Verification items for the finished model (mm, model axes). A direction names the side the tool comes from. Give positions to 0.01 mm unless a question says otherwise; leave off trailing zeros. Write each loop counter-clockwise with the first axis right and the second up, starting at its lowest first coordinate (ties: lowest second). Pieces come first, ordered by that corner, then holes.
from build123d import *

# Parameters (mm, degrees)
SKETCH1_W                       = 8
SKETCH1_H                       = 15
FIRST_CHAMBER_BLOCK_DEPTH       = 15
SKETCH2_W                       = 6
SKETCH2_H                       = 11
FIRST_CHAMBER_CAVITY_DEPTH      = 13
SKETCH3_W                       = 15
SKETCH3_H                       = 3
CHAMBER_SPACER_DEPTH            = 2
PATTERN_CHAMBERS_COUNT          = 11
PATTERN_CHAMBERS_PITCH          = 10
SKETCH4_W                       = 15
SKETCH4_H                       = 12
THICKEN_END_1_DEPTH             = 2
SKETCH5_W                       = 15
SKETCH5_H                       = 15
THICKEN_END_2_DEPTH             = 2
SKETCH6_W                       = 94
SKETCH6_H                       = 2
CENTRAL_AIR_CHANNEL_DEPTH       = 2
SKETCH7_W                       = 108
SKETCH7_H                       = 13
SKETCH7_W_2                     = 106
SKETCH7_H_2                     = 11
BONDING_RIDGE_DEPTH             = 2
SKETCH9_W                       = 2
SKETCH9_H                       = 2.5
BONDING_BUMPS_DEPTH             = 2
PATTERN_BONDING_BUMPS_COUNT     = 10
PATTERN_BONDING_BUMPS_PITCH     = 10
SKIZZE1_W                       = 112
SKIZZE1_H                       = 15
SCHNITT_LINEAR_AUSTRAGEN1_DEPTH = 113.026782512
SKIZZE2_W                       = 2
SKIZZE2_H                       = 1
AUFSATZ_LINEAR_AUSTRAGEN1_DEPTH = 9
LINEARES_MUSTER1_COUNT          = 10
LINEARES_MUSTER1_PITCH          = 10
SKIZZE4_R                       = 1.25
SCHNITT_LINEAR_AUSTRAGEN3_DEPTH = 112.776562839


with BuildPart() as part:
    # Sketch1 → first chamber block (new body)
    with BuildSketch(Plane.XY):
        with Locations((4, 7.5)):
            Rectangle(SKETCH1_W, SKETCH1_H)
    extrude(amount=FIRST_CHAMBER_BLOCK_DEPTH)

    # Sketch2 → first chamber cavity (cut)
    with BuildSketch(Plane.XZ):
        with Locations((4, 7.5)):
            Rectangle(SKETCH2_W, SKETCH2_H)
    extrude(amount=-FIRST_CHAMBER_CAVITY_DEPTH, mode=Mode.SUBTRACT)

    # Sketch3 → chamber spacer (add)
    with BuildSketch(Plane(origin=(8, 0, 0), x_dir=(0, 0, -1), z_dir=(1, 0, 0))):
        with Locations((-7.5, 1.5)):
            Rectangle(SKETCH3_W, SKETCH3_H)
    extrude(amount=CHAMBER_SPACER_DEPTH)


with BuildPart() as pattern_chambers_1:
    # pattern chambers: pattern copy
    add(part.part.moved(Location(Vector(1, 0, 0) * (1 * PATTERN_CHAMBERS_PITCH))))


with BuildPart() as pattern_chambers_2:
    # pattern chambers: pattern copy
    add(part.part.moved(Location(Vector(1, 0, 0) * (2 * PATTERN_CHAMBERS_PITCH))))


with BuildPart() as pattern_chambers_3:
    # pattern chambers: pattern copy
    add(part.part.moved(Location(Vector(1, 0, 0) * (3 * PATTERN_CHAMBERS_PITCH))))


with BuildPart() as pattern_chambers_4:
    # pattern chambers: pattern copy
    add(part.part.moved(Location(Vector(1, 0, 0) * (4 * PATTERN_CHAMBERS_PITCH))))


with BuildPart() as pattern_chambers_5:
    # pattern chambers: pattern copy
    add(part.part.moved(Location(Vector(1, 0, 0) * (5 * PATTERN_CHAMBERS_PITCH))))


with BuildPart() as pattern_chambers_6:
    # pattern chambers: pattern copy
    add(part.part.moved(Location(Vector(1, 0, 0) * (6 * PATTERN_CHAMBERS_PITCH))))


with BuildPart() as pattern_chambers_7:
    # pattern chambers: pattern copy
    add(part.part.moved(Location(Vector(1, 0, 0) * (7 * PATTERN_CHAMBERS_PITCH))))


with BuildPart() as pattern_chambers_8:
    # pattern chambers: pattern copy
    add(part.part.moved(Location(Vector(1, 0, 0) * (8 * PATTERN_CHAMBERS_PITCH))))


with BuildPart() as pattern_chambers_9:
    # pattern chambers: pattern copy
    add(part.part.moved(Location(Vector(1, 0, 0) * (9 * PATTERN_CHAMBERS_PITCH))))


with BuildPart() as pattern_chambers_10:
    # pattern chambers: pattern copy
    add(part.part.moved(Location(Vector(1, 0, 0) * (10 * PATTERN_CHAMBERS_PITCH))))

    # combine into 1 solid body: union pattern chambers_9, pattern chambers_8, pattern chambers_7, pattern chambers_6, pattern chambers_5, pattern chambers_4, pattern chambers_3, pattern chambers_2, pattern chambers_1, part
    add(pattern_chambers_9.part)
    add(pattern_chambers_8.part)
    add(pattern_chambers_7.part)
    add(pattern_chambers_6.part)
    add(pattern_chambers_5.part)
    add(pattern_chambers_4.part)
    add(pattern_chambers_3.part)
    add(pattern_chambers_2.part)
    add(pattern_chambers_1.part)
    add(part.part)

    # Sketch4 → thicken end 1 (add)
    with BuildSketch(Plane(origin=(108, 0, 0), x_dir=(0, 0, -1), z_dir=(1, 0, 0))):
        with Locations((-7.5, 9)):
            Rectangle(SKETCH4_W, SKETCH4_H)
    extrude(amount=THICKEN_END_1_DEPTH)

    # Sketch5 → thicken end 2 (add)
    with BuildSketch(Plane.ZY):
        with Locations((7.5, 7.5)):
            Rectangle(SKETCH5_W, SKETCH5_H)
    extrude(amount=THICKEN_END_2_DEPTH)

    # Sketch6 → central air channel (cut)
    with BuildSketch(Plane.XZ):
        with Locations((54, 7.5)):
            Rectangle(SKETCH6_W, SKETCH6_H)
    extrude(amount=-CENTRAL_AIR_CHANNEL_DEPTH, mode=Mode.SUBTRACT)

    # Sketch7 → bonding ridge (add)
    with BuildSketch(Plane.XZ):
        with Locations((54, 7.5)):
            Rectangle(SKETCH7_W, SKETCH7_H)
        with Locations((54, 7.5)):
            Rectangle(SKETCH7_W_2, SKETCH7_H_2, mode=Mode.SUBTRACT)
    extrude(amount=BONDING_RIDGE_DEPTH)

    # Sketch9 → bonding bumps (add)
    with BuildSketch(Plane.XZ):
        with Locations((9, 10.75)):
            Rectangle(SKETCH9_W, SKETCH9_H)
        with Locations((9, 4.25)):
            Rectangle(SKETCH9_W, SKETCH9_H)
    bonding_bumps = extrude(amount=BONDING_BUMPS_DEPTH)

    # pattern bonding bumps: bonding bumps ×10
    with Locations(*[(i * PATTERN_BONDING_BUMPS_PITCH, 0, 0) for i in range(1, PATTERN_BONDING_BUMPS_COUNT)]):
        add(bonding_bumps)

    # Skizze1 → Schnitt-Linear austragen1 (cut, through all)
    with BuildSketch(Plane.XZ):
        with Locations((54, 7.5)):
            Rectangle(SKIZZE1_W, SKIZZE1_H)
    extrude(amount=SCHNITT_LINEAR_AUSTRAGEN1_DEPTH, mode=Mode.SUBTRACT)

    # Skizze2 → Aufsatz-Linear austragen1 (add)
    with BuildSketch(Plane(origin=(0, 3, 0), x_dir=(1, 0, 0), z_dir=(0, 1, 0))):
        with Locations((99, -0.5)):
            Rectangle(SKIZZE2_W, SKIZZE2_H)
        with Locations((99, -14.5)):
            Rectangle(SKIZZE2_W, SKIZZE2_H)
    aufsatz_linear_austragen1 = extrude(amount=AUFSATZ_LINEAR_AUSTRAGEN1_DEPTH)

    # Lineares Muster1: Aufsatz-Linear austragen1 ×10
    with Locations(*[(-i * LINEARES_MUSTER1_PITCH, 0, 0) for i in range(1, LINEARES_MUSTER1_COUNT)]):
        add(aufsatz_linear_austragen1)

    # Skizze4 → Schnitt-Linear austragen3 (cut, through all)
    with BuildSketch(Plane.XY.offset(2)):
        with Locations((4, 6.5)):
            Circle(SKIZZE4_R)
    extrude(amount=-SCHNITT_LINEAR_AUSTRAGEN3_DEPTH, mode=Mode.SUBTRACT)


solid = pattern_chambers_10.part
Item 1: Release check for a two-part mould opening along X. For faces 4 (the face through (110, 8, 8)), 5 (the face through (34, 15, 7)), 6 (the face through (57, 6, 7)) record: released by +X, released by -X, zero draft, split by the parting line, or undercut.
Answer key:
face 4: released by +X
face 5: zero draft
face 6: undercut
Item 2: Set-up check for faces 1 (the face through (49, 7, 1)), 2 (the face through (14, 13, 8)), 3 (the face through (64, 15, 7)): record each of +Z, -Z, +X, -X, +Y, -Y from which the full face is reachable in a straight line by a thin tool's end or side.
Answer key:
face 1: +Y
face 2: -Y
face 3: +Z, -Z, +X, -X, +Y
Item 3: Depth check by flat-ended pin: pin 1 (3 mm diameter, centred on x = 74, y = 2.5, fed in from -Z); pin 2 (1.6 mm diameter, centred on x = 78.5, z = 7.5, fed in from -Y); pin 3 (0.5 mm diameter, centred on x = 19, z = 14.5, fed in from +Y). Enter the tip coordinate at first touch or a pass-through.
Answer key:
pin 1: stops at z = 0
pin 2: stops at y = 2
pin 3: stops at y = 12
Item 4: Scan lines: line 1 along Y through (x, z) = (4, 1.25); line 2 along X through (y, z) = (1.75, 8.25); line 3 along Z through (x, y) = (26, 8.25). Record each from-to range of solid material in increasing order.
Answer key:
line 1: y = 0 to 5.25, 7.75 to 15
line 2: x = -2 to 1, 107 to 110
line 3: z = 0 to 2, 13 to 15
Item 5: Sectioned sample at C-C on x = 102. Record the cut outline in (y, z).
Answer key:
outline: (0, 0) - (15, 0) - (15, 15) - (0, 15) - (0, 13) - (13, 13) - (13, 2) - (0, 2) - close
Item 6: Sectioned sample at A-A on x = 4. Record the cut outline in (y, z), then the cut area to 3 significant figures.
Answer key:
outline: (0, 0) - (5.25, 0) - (5.25, 2) - (0, 2) - close; (0, 13) - (13, 13) - (13, 2) - (7.75, 2) - (7.75, 0) - (15, 0) - (15, 15) - (0, 15) - close
area: 77.0 mm2
Item 7: Sectioned sample at B-B on y = 6.5. State how many separate pieces and enclosed holes the cut face has, then the cut area to 3 significant figures.
Answer key:
separate pieces: 1
enclosed holes: 20
area: 689 mm2
